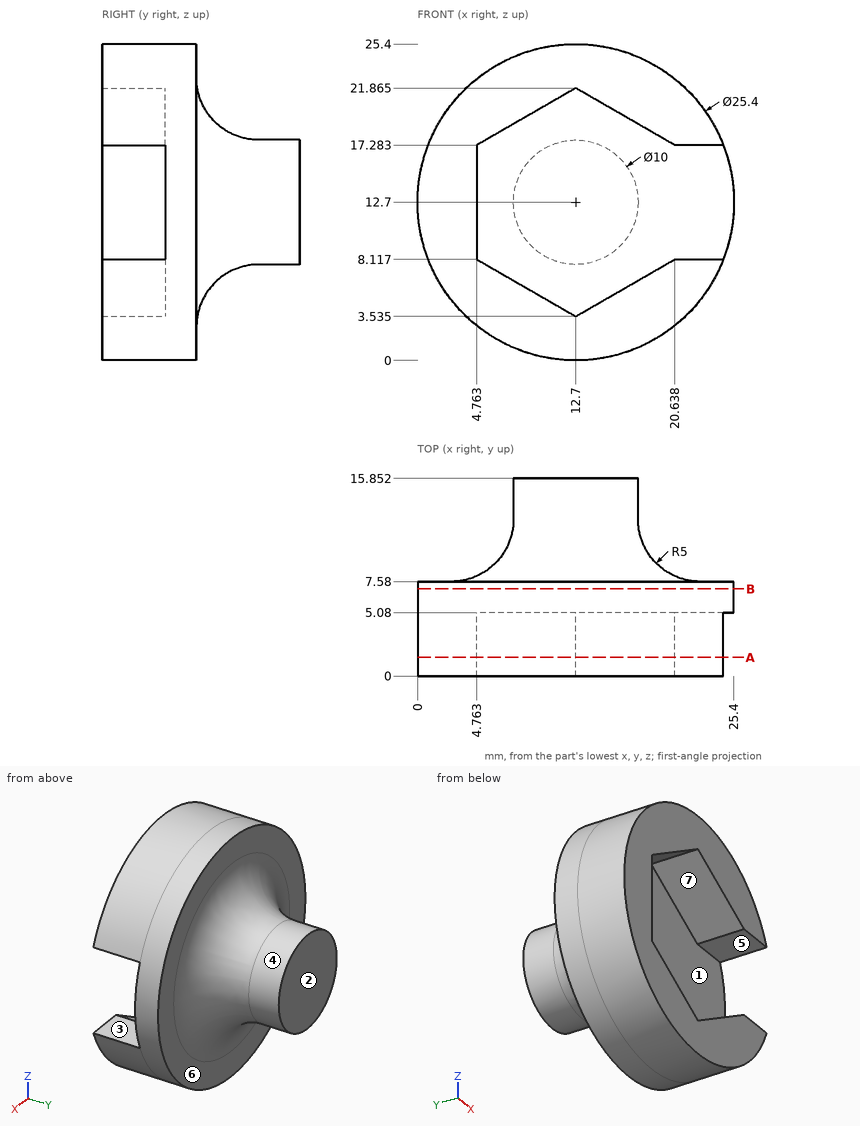
Here's the drawing with two shaded views (mm, measured from the low corner). I have some questions. A direction names the side the tool comes from. Give positions to 0.01 mm unless a question says otherwise; leave off trailing zeros. Write each loop counter-clockwise with the first axis right and the second up, starting at its lowest first coordinate (ties: lowest second). Pieces come first, ordered by that corner, then holes. Notation, with made-up numbers: (-11, 49) -> (39, 49) arc R13 cw to (39, 64) -> close; hole circle Ø11 at (-20, 85). An arc over 180 degrees is marked (long way). One line per item, written item: value.
Q1. Imagine slicing it at A-A on y = 1.5. Please give me the cut outline in (x, z) (1 decimal).
Results found:
outline: (4.8, 8.1) -> (4.8, 17.3) -> (12.7, 21.9) -> (20.6, 17.3) -> (24.5, 17.3) arc R12.7 ccw (long way) to (24.5, 8.1) -> (20.6, 8.1) -> (12.7, 3.5) -> close
Q2. Please list where these lines run through material, in increasing order: line 1 (Y direction, x = 4.25, z = 5.75); line 2 (Y direction, x = 15.25, z = 12.25); line 3 (Z direction, x = 17, y = 3). Write a range as [from, to].
Results found:
line 1: y = [0, 7.58]
line 2: y = [5.08, 15.85]
line 3: z = [0.75, 6.02], [19.38, 24.65]
Q3. Imagine slicing it at B-B on y = 7. Please give me the cut outline in (x, z), and give its area (3 significant figures).
Results found:
outline: circle Ø25.4 at (12.7, 12.7)
area: 507 mm^2
Q4. Which directions (+Z, -Z, +X, -X, +Y, -Y) give clear straight access to the entire face, cutting with the end or side of a thin tool? Please do the marked faces 5, 6 and 7.
Results found:
face 5: +X, -Y
face 6: +Y
face 7: -Y
Q5. For P1, Ø12, axis at x = 15.5, z = 17, coming from the -Y side; P2, Ø1.5, axis at y = 2, z = 22, coming from the -X side; P3, Ø5, axis at y = 4.5, z = 3.5, coming from the +X side; P4, Ø5.5, axis at y = 2.5, z = 11.5, coming from the +X side, each with a flat end and sliding along its axis, tell me the tip position at first contact or that it passes through.
Results found:
P1: stops at y = 0
P2: stops at x = 3.31
P3: stops at x = 23.49
P4: stops at x = 25.4
Q6. We'd pull the mould along Z, two halves only. Please class the marked faces 1, 2, 3 and 4: +Z half, -Z half, draft (parallel to the pull), parting line (faces both ways), or undercut.
Results found:
face 1: undercut
face 2: draft
face 3: undercut
face 4: parting line
